Work out the finished part from the listing and answer in its coordinate system (mm). A direction names the side the tool comes from. Give positions to 0.01 mm unless a question says otherwise; leave off trailing zeros. Loops run counter-clockwise (first coordinate to the right, second up) from the corner with the lowest first, then second, coordinate; pieces in that order, holes last. Notation, with made-up numbers: (55, 89) - (70, 89) arc R10 cw to (70, 105) - close; hole circle Ø9 at (-32.5, -21). An arc over 180 degrees is marked (long way). One line per item, written item: value.
from build123d import *

# Parameters (mm, degrees)
F0_W      = 145.814352
F0_H      = 97.318382
F0_W_2    = 133.114352
F0_H_2    = 84.618382
F1_DEPTH  = 25.4
F0_R      = 10.988187
F2_DEPTH  = 2.286
F0_R_2    = 3.402604
F3_DEPTH  = 25.4
F4_DEPTH  = 25.4
F5_DEPTH  = 25.4
F6_R      = 5.08
F7_R      = 5.08
F8_R      = 5.08
F9_R      = 5.08
F10_R     = 5.08
F11_R     = 5.08
F12_R     = 5.08
F13_DEPTH = 27.94


with BuildPart() as f1:
    # F0 (on Top) → F1 (new body)
    with BuildSketch(Plane.XY):
        Rectangle(F0_W, F0_H)
        Rectangle(F0_W_2, F0_H_2, mode=Mode.SUBTRACT)
    extrude(amount=F1_DEPTH)

    # F0 (on Top) → F2 (join)
    with BuildSketch(Plane.XY):
        Rectangle(F0_W_2, F0_H_2)
        with Locations((-52.712649, -30.396467)):
            Circle(F0_R, mode=Mode.SUBTRACT)
        with Locations((52.712649, -30.396467)):
            Circle(F0_R, mode=Mode.SUBTRACT)
        with Locations((-52.712649, 30.396467)):
            Circle(F0_R, mode=Mode.SUBTRACT)
        with Locations((52.712649, 30.396467)):
            Circle(F0_R, mode=Mode.SUBTRACT)
    extrude(amount=F2_DEPTH)

    # F0 (on Top) → F3 (join)
    with BuildSketch(Plane.XY):
        with Locations((-52.712649, 30.396467)):
            Circle(F0_R)
        with Locations((-52.712649, 30.396467)):
            Circle(F0_R_2, mode=Mode.SUBTRACT)
    extrude(amount=F3_DEPTH)

    # F0 (on Top) → F4 (join)
    with BuildSketch(Plane.XY):
        with Locations((52.712649, 30.396467)):
            Circle(F0_R)
        with Locations((52.712649, 30.396467)):
            Circle(F0_R_2, mode=Mode.SUBTRACT)
    extrude(amount=F4_DEPTH)

    # F0 (on Top) → F5 (join)
    with BuildSketch(Plane.XY):
        with Locations((-52.712649, -30.396467)):
            Circle(F0_R)
        with Locations((-52.712649, -30.396467)):
            Circle(F0_R_2, mode=Mode.SUBTRACT)
        with Locations((52.712649, -30.396467)):
            Circle(F0_R)
        with Locations((52.712649, -30.396467)):
            Circle(F0_R_2, mode=Mode.SUBTRACT)
    extrude(amount=F5_DEPTH)

    # F6
    f6_edges = [f1.edges().sort_by_distance(p)[0] for p in [
        (-72.907176, -48.659191, 12.7),
        (72.907176, -48.659191, 12.7),
    ]]
    fillet(f6_edges, radius=F6_R)

    # F7
    f7_edges = [f1.edges().sort_by_distance(p)[0] for p in [
        (-66.557176, 42.309191, 13.843),
    ]]
    fillet(f7_edges, radius=F7_R)

    # F8
    f8_edges = [f1.edges().sort_by_distance(p)[0] for p in [
        (72.907176, 48.659191, 12.7),
    ]]
    fillet(f8_edges, radius=F8_R)

    # F9
    f9_edges = [f1.edges().sort_by_distance(p)[0] for p in [
        (-72.907176, 48.659191, 12.7),
    ]]
    fillet(f9_edges, radius=F9_R)

    # F10
    f10_edges = [f1.edges().sort_by_distance(p)[0] for p in [
        (66.557176, -42.309191, 13.843),
    ]]
    fillet(f10_edges, radius=F10_R)

    # F11
    f11_edges = [f1.edges().sort_by_distance(p)[0] for p in [
        (66.557176, 42.309191, 13.843),
    ]]
    fillet(f11_edges, radius=F11_R)

    # F12
    f12_edges = [f1.edges().sort_by_distance(p)[0] for p in [
        (-66.557176, -42.309191, 13.843),
    ]]
    fillet(f12_edges, radius=F12_R)

    # F1_face (on face) → F13 (join)
    with BuildSketch(Plane.XY.offset(25.4)):
        with BuildLine():
            Line((67.827176, 48.659191), (-67.827176, 48.659191))
            ThreePointArc((-67.827176, 48.659191), (-71.419279, 47.171294), (-72.907176, 43.579191))
            Line((-72.907176, 43.579191), (-72.907176, -43.579191))
            ThreePointArc((-72.907176, -43.579191), (-71.419279, -47.171294), (-67.827176, -48.659191))
            Line((-67.827176, -48.659191), (67.827176, -48.659191))
            ThreePointArc((67.827176, -48.659191), (71.419279, -47.171294), (72.907176, -43.579191))
            Line((72.907176, -43.579191), (72.907176, 43.579191))
            ThreePointArc((72.907176, 43.579191), (71.419279, 47.171294), (67.827176, 48.659191))
        make_face()
        with BuildLine():
            Line((61.477176, -42.309191), (-61.477176, -42.309191))
            ThreePointArc((-61.477176, -42.309191), (-65.069279, -40.821294), (-66.557176, -37.229191))
            Line((-66.557176, -37.229191), (-66.557176, 37.229191))
            ThreePointArc((-66.557176, 37.229191), (-65.069279, 40.821294), (-61.477176, 42.309191))
            Line((-61.477176, 42.309191), (61.477176, 42.309191))
            ThreePointArc((61.477176, 42.309191), (65.069279, 40.821294), (66.557176, 37.229191))
            Line((66.557176, 37.229191), (66.557176, -37.229191))
            ThreePointArc((66.557176, -37.229191), (65.069279, -40.821294), (61.477176, -42.309191))
        make_face(mode=Mode.SUBTRACT)
    extrude(amount=F13_DEPTH)


solid = f1.part
1. Section A-A (z = 18) is taken. Count the separate pieces of the cut face and the enclosed holes in it, and give its area (3 significant figures).
Output:
separate pieces: 5
enclosed holes: 5
area: 4,300 mm²
2. Find the intervals of material crossed by line 1 along X through (y, z) = (-19, 45); line 2 along X through (y, z) = (30.5, 4); line 3 along Y through (x, z) = (44.5, 34.5), in increasing order.
Output:
line 1: x = -72.91 to -66.56, 66.56 to 72.91
line 2: x = -72.91 to -66.56, -63.7 to -56.11, -49.31 to -41.72, 41.72 to 49.31, 56.11 to 63.7, 66.56 to 72.91
line 3: y = -48.66 to -42.31, 42.31 to 48.66
3. Flat-ended cylindrical pins translate along their axes: pin 1 Ø6.5 at (x, y) = (-49, -29) entering from +Z; pin 2 Ø12 at (x, y) = (-19.5, -6.5) entering from +Z. Find the tip coordinate at first contact, or state that the pin passes through.
Output:
pin 1: stops at z = 25.4
pin 2: stops at z = 2.29
4. For faces 1 (the flat face through (-1, 1, 0)), 2 (the flat face through (-1, 42.309, 27)), determine the directions among +Z, -Z, +X, -X, +Y, -Y from which every point of the face is accessible in a straight line to the end or side of a thin tool.
Output:
face 1: -Z, +X, -X, +Y, -Y
face 2: +Z
5. Section D-D (x = 17) is taken. Write down the section's boundary in (y, z), and give its area (3 significant figures).
Output:
outline: (-48.66, 0) - (48.66, 0) - (48.66, 53.34) - (42.31, 53.34) - (42.31, 2.29) - (-42.31, 2.29) - (-42.31, 53.34) - (-48.66, 53.34) - close
area: 871 mm²
6. The mould has two halves that part along X. Classify faces 3 (the flat face through (1, 48.659, 26)), 4 (the flat face through (-66.557, -1, 27)), 5 (the cylindrical face through (-71.38, 47.21, 12.88)), 6 (the flat face through (1, -42.309, 27)): released by +X, released by -X, zero draft, split by the parting line, or undercut.
Output:
face 3: zero draft
face 4: undercut
face 5: released by -X
face 6: undercut
7. Section B-B (z = 35.5) is taken. Write down the section's boundary in (x, y), and give its area (3 significant figures).
Output:
outline: (-72.91, -43.58) arc R5.08 ccw to (-67.83, -48.66) - (67.83, -48.66) arc R5.08 ccw to (72.91, -43.58) - (72.91, 43.58) arc R5.08 ccw to (67.83, 48.66) - (-67.83, 48.66) arc R5.08 ccw to (-72.91, 43.58) - close; hole (-66.56, -37.23) arc R5.08 ccw to (-61.48, -42.31) - (61.48, -42.31) arc R5.08 ccw to (66.56, -37.23) - (66.56, 37.23) arc R5.08 ccw to (61.48, 42.31) - (-61.48, 42.31) arc R5.08 ccw to (-66.56, 37.23) - close
area: 2,930 mm²
8. Section C-C (y = 12) is taken. Write down the section's boundary in (x, z).
Output:
outline: (-72.91, 0) - (72.91, 0) - (72.91, 53.34) - (66.56, 53.34) - (66.56, 2.29) - (-66.56, 2.29) - (-66.56, 53.34) - (-72.91, 53.34) - close
